Answer from the drawing. Dimensions are ordinates in mm from the lowest x, y and z of the part. Coordinates: 2 decimals unless noted, no trailing zeros. Order: outer loops, then holes, each group sorted by start corner. A loop starts at its lowest first (then second) coordinate and runs counter-clockwise, first axis right, second up. Notation, with made-up numbers: (15, 36.25) - (72, 36.25) arc R13 cw to (72, 42.25) - close; hole circle Ø10 at (7.5, 10). An arc over 180 degrees is marked (long way). Answer as a JSON object with one key per item and string values. Group by question number.
1) This flat-tipped pin is pushed along its axis until it touches: P1, Ø2, axis at y = 2.5, z = 1, coming from the +X side. Where does it stop, or does it pass through?
2) Find the intervals of material crossed by line 1 along X through (y, z) = (6, 5.25); line 2 along X through (y, z) = (7, 3.75), in increasing order.
3) Section A-A (z = 2) is taken. Give the vertices of the cut face in (x, y).
4) Section B-B (y = 2.25) is taken. Give the vertices of the cut face in (x, z), plus the area to 3 significant figures.
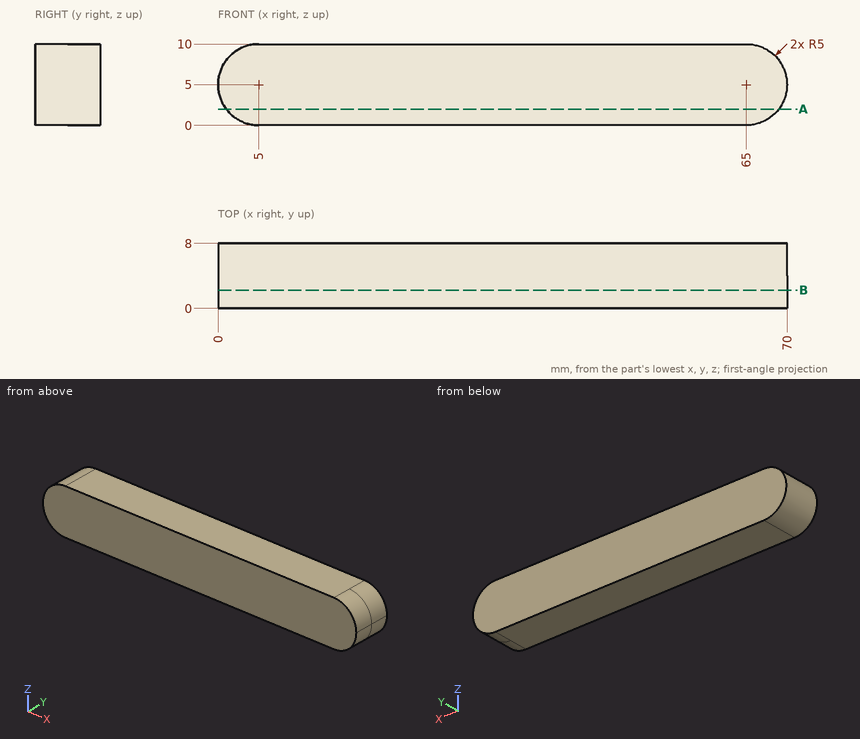
Report:
{
 "1": {"P1": "stops at x = 69"},
 "2": {"line 1": "x = 0.01 to 69.99", "line 2": "x = 0.16 to 69.84"},
 "3": {"outline": "(1, 0) - (69, 0) - (69, 8) - (1, 8) - close"},
 "4": {"outline": "(5, 0) - (65, 0) arc R5 ccw to (65, 10) - (5, 10) arc R5 ccw to start", "area": "679 mm²"}
}
